Geometry: final body of the model. Coordinates: model frame, mm. Coordinates: 2 decimals unless noted, no trailing zeros. Order: outer loops, then holes, each group sorted by start corner. A loop starts at its lowest first (then second) coordinate and runs counter-clockwise, first axis right, second up. Notation, with made-up numbers: M -17.5,-6.5 L 16.5,-6.5 A23 ccw 16.5,19.5 Z; hole C 28.5,-21.75 d6. An arc over 180 degrees is marked long. Write item = value, one per line.
Autodesk Inventor part; units mm, degrees
ref_plane "YZ Plane" through (0, 0, 0) normal (1, 0, 0) x (0, 1, 0)
ref_plane "XZ Plane" through (0, 0, 0) normal (0, 1, 0) x (-1, 0, 0)
ref_plane "XY Plane" through (0, 0, 0) normal (0, 0, 1) x (1, 0, 0)
sketch "Sketch1" plane through (0, 0, 0) normal (1, 0, 0) x (0, 1, 0)
  line L0 (64.7557, 308.0174) -> (-36.8443, 308.0174)
  line L1 (-36.8443, 308.0174) -> (-36.8443, -314.2826)
  line L2 (-36.8443, -314.2826) -> (64.7557, -314.2826)
  line L3 (64.7557, -314.2826) -> (64.7557, 308.0174)
  dimension "d2" = 622.3
  dimension "d3" = 101.6
extrude "Board" add sketch "Sketch1" along normal blind 19.05
sketch "Sketch8" plane through (19.05, 0, 0) normal (1, 0, 0) x (0, 0, -1)
  line L0 (-308.0174, 55.2307) -> (314.2826, 55.2307)
  line L1 (314.2826, 55.2307) -> (314.2826, 45.7057)
  line L2 (314.2826, 45.7057) -> (-308.0174, 45.7057)
  line L3 (-308.0174, 45.7057) -> (-308.0174, 55.2307)
  line L4 (-308.0174, 64.7557) -> (-308.0174, -36.8443)
  line L5 (314.2826, -36.8443) -> (314.2826, 64.7557)
  line L6 (314.2826, 64.7557) -> (-308.0174, 64.7557)
  point P0 (0, 0)
  dimension "d22" = 9.525
  dimension "d23" = 9.525
extrude "Lenghtwise Dado for Base" cut sketch "Sketch8" against normal blind 9.525 contours L0 L1 L2 L3
sketch "Sketch 9" plane through (0, 64.7557, 308.0174) normal (0, 1, 0) x (1, 0, 0)
  line L0 (19.05, 0) -> (9.525, 0)
  line L1 (9.525, 0) -> (9.525, 454.025)
  line L2 (9.525, 454.025) -> (19.05, 454.025)
  line L3 (19.05, 454.025) -> (19.05, 0)
  line L4 (19.05, 622.3) -> (19.05, 0)
  line L5 (0, 622.3) -> (19.05, 622.3)
  line L6 (0, 0) -> (19.05, 0)
  point P0 (0, 308.0174)
  dimension "d26" = 454.025
  dimension "d27" = 9.525
extrude "Lengthwise stop dado for Sides" cut sketch "Sketch 9" against normal blind 9.525
sketch "Sketch12" plane through (19.05, 0, 0) normal (1, 0, 0) x (0, 0, -1)
  line L0 (-308.0174, 26.6557) -> (314.2826, 26.6557)
  line L1 (314.2826, 26.6557) -> (314.2826, 45.7057)
  line L2 (314.2826, 45.7057) -> (-308.0174, 45.7057)
  line L3 (-308.0174, 45.7057) -> (-308.0174, 26.6557)
  line L4 (314.2826, 45.7057) -> (-308.0174, 45.7057)
  line L5 (-308.0174, 45.7057) -> (-308.0174, -36.8443)
  line L6 (314.2826, -36.8443) -> (314.2826, 45.7057)
  point P0 (0, 0)
  dimension "d30" = 19.05
extrude "Lenghtwise full dado for base" cut sketch "Sketch12" against normal blind 9.525
properties part number "Base Runner Side Right"
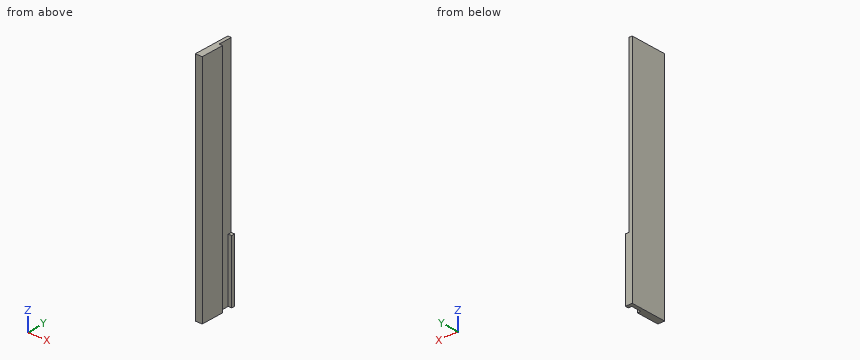
1) Pin query (flat end, axial travel): pin 1 (3 mm diameter, centred on x = 14, z = 57.5, fed in from +Y); pin 2 (5 mm diameter, centred on x = 13.5, y = 59.5, fed in from +Z). Return the tip coordinate at first contact, or that it passes through.
Numbers:
pin_1 = 26.66
pin_2 = -146.01
2) Section A-A, the plane x = 12.75. Return loops of the section in (y, z), and give its area (3 significant figures).
Numbers:
outline = M -36.84,-314.28 L 26.66,-314.28 L 26.66,308.02 L -36.84,308.02 Z; M 55.23,-314.28 L 64.76,-314.28 L 64.76,-146.01 L 55.23,-146.01 Z
area = 41,100 mm²
3) Section C-C, the plane y = 46. Return loops of the section in (x, z) (3 decimals).
Numbers:
outline = M 0,-314.283 L 9.525,-314.283 L 9.525,308.017 L 0,308.017 Z
4) Section D-D, the plane z = -107.5. Return loops of the section in (x, y) (3 decimals), and give its area (3 significant figures).
Numbers:
outline = M 0,-36.844 L 19.05,-36.844 L 19.05,26.656 L 9.525,26.656 L 9.525,64.756 L 0,64.756 Z
area = 1,570 mm²
5) Section B-B, the plane z = -205. Return loops of the section in (x, y) (3 decimals), and give its area (3 significant figures).
Numbers:
outline = M 0,-36.844 L 19.05,-36.844 L 19.05,26.656 L 9.525,26.656 L 9.525,55.231 L 19.05,55.231 L 19.05,64.756 L 0,64.756 Z
area = 1,660 mm²
6) Line query: L1, parallel to Y at x = 16.75, z = -175; L2, parallel to Z at x = 15.5, y = 59.5; L3, parallel to X at y = 51, z = 71.5 (3 decimals). Output: solid intervals per line, ascending.
Numbers:
L1 = -36.84 to 26.66, 55.23 to 64.76
L2 = -314.28 to -146.01
L3 = 0 to 9.525
